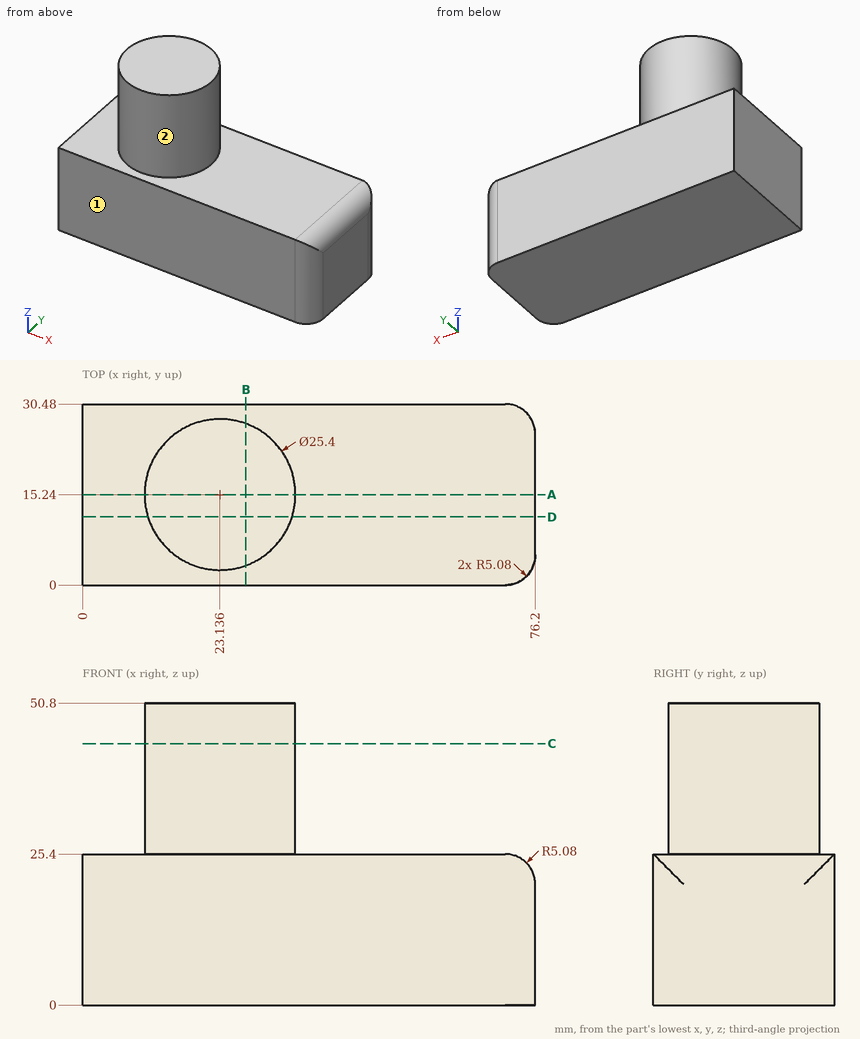
Part print with two shaded views. Sizes in mm from the minimum x, y, z corner. A direction names the side the tool comes from. Give positions to 0.01 mm unless a question says otherwise; leave off trailing zeros. Order: outer loops, then holes, each group sorted by start corner. A loop starts at its lowest first (then second) coordinate and runs counter-clockwise, first axis right, second up. Notation, with made-up numbers: M 44,-10.75 L 68,-10.75 A27 ccw 68,18.25 Z; hole C 89,40.5 d11. An arc over 180 degrees is marked long. Put each result on its own line as item: value.
Item 1: Which spindle directions (+Z, -Z, +X, -X, +Y, -Y) get a long thin tool onto all of the face, cutting with end or side? Do the marked faces 1 and 2. Say none if no direction does.
Results are:
face 1: +Z, -Z, +X, -X, -Y
face 2: +Z
Item 2: Cut at A-A on y = 15.24. Write the cut outline in (x, z).
Results are:
outline: M 0,0 L 76.2,0 L 76.2,20.32 A5.08 ccw 71.12,25.4 L 35.84,25.4 L 35.84,50.8 L 10.44,50.8 L 10.44,25.4 L 0,25.4 Z
Item 3: Cut at B-B on x = 27.5. Write the cut outline in (y, z).
Results are:
outline: M 0,0 L 30.48,0 L 30.48,25.4 L 27.17,25.4 L 27.17,50.8 L 3.31,50.8 L 3.31,25.4 L 0,25.4 Z
Item 4: Drop flat-ended pins along their axis: pin 1 Ø1 at (y, z) = (9.5, 44.5) entering from +X (1 decimal); pin 2 Ø1.5 at (x, y) = (30.5, 27.5) entering from +Z. Give the stop position or say it passes through.
Results are:
pin 1: x = 34.7
pin 2: z = 25.4
Item 5: Cut at C-C on z = 44. Write the cut outline in (x, y), then the cut area to 3 significant figures.
Results are:
outline: C 23.14,15.24 d25.4
area: 507 mm2
Item 6: Wall check: probe 1 along Z at (x, y) = (12, 8.5); probe 2 along X at (y, z) = (15, 29); probe 3 along X at (y, z) = (3.5, 18.5). Give the ranges that are in metal, low to high.
Results are:
probe 1: 0 to 25.4
probe 2: 10.44 to 35.83
probe 3: 0 to 75.95
Item 7: Cut at D-D on y = 11.5. Write the cut outline in (x, z).
Results are:
outline: M 0,0 L 76.2,0 L 76.2,20.32 A5.08 ccw 71.12,25.4 L 35.27,25.4 L 35.27,50.8 L 11,50.8 L 11,25.4 L 0,25.4 Z
